from build123d import *

# Parameters (mm, degrees)
BOSS_EXTRUDE1_DEPTH = 247.65
FILLET2_R           = 0.254
FILLET1_R           = 1.27
SKETCH5_W           = 7.112
SKETCH5_H           = 2.54
BOSS_EXTRUDE2_DEPTH = 495.3


with BuildPart() as part:
    # Sketch3 → Boss-Extrude1 (new body, symmetric)
    with BuildSketch(Plane.XY):
        with BuildLine():
            Line((-12.7, 12.7), (-1.796051224, 1.796051224))
            ThreePointArc((-1.796051224, 1.796051224), (-0.972015918, 2.346654013), (0, 2.54))
            Line((0, 2.54), (0, 4.826))
            Line((0, 4.826), (-1.977846327, 4.826))
            ThreePointArc((-1.977846327, 4.826), (-2.949862246, 5.019345987), (-3.773897552, 5.569948776))
            Line((-3.773897552, 5.569948776), (-7.772528286, 9.56857951))
            ThreePointArc((-7.772528286, 9.56857951), (-7.847628361, 9.946133082), (-7.527553898, 10.16))
            Line((-7.527553898, 10.16), (-3.302, 10.16))
            Line((-3.302, 10.16), (-3.302, 12.7))
            Line((-3.302, 12.7), (-12.7, 12.7))
        make_face()
    extrude(amount=BOSS_EXTRUDE1_DEPTH, both=True)

    # Fillet2
    fillet2_edges = [part.edges().sort_by_distance(p)[0] for p in [
        (-3.302, 12.7, 0),
        (-3.302, 10.16, 0),
    ]]
    fillet(fillet2_edges, radius=FILLET2_R)

    # Mirror1: part across plane


with BuildPart() as part_1:
    add(part.part)
    add(part.part.mirror(Plane(origin=(0, 0, 247.65), x_dir=(0, 0, 1), z_dir=(0.707106781, 0.707106781, 0))))

    # Fillet1
    fillet1_edges = [part_1.edges().sort_by_distance(p)[0] for p in [
        (-12.7, 12.7, 0),
    ]]
    fillet(fillet1_edges, radius=FILLET1_R)

    # Mirror2: part across plane


with BuildPart() as part_2:
    add(part_1.part)
    add(part_1.part.mirror(Plane(origin=(0, 0, 247.65), x_dir=(0, 0, 1), z_dir=(0, 1, 0))))

    # Mirror5: part across plane


with BuildPart() as part_3:
    add(part_2.part)
    add(part_2.part.mirror(Plane(origin=(0, 0, 247.65), x_dir=(0, 0, 1), z_dir=(-1, 0, 0))))

    # Sketch5 → Boss-Extrude2 (add, through all)
    with BuildSketch(Plane.XY.offset(247.65)):
        with Locations((0, -11.43)):
            Rectangle(SKETCH5_W, SKETCH5_H)
    extrude(amount=-BOSS_EXTRUDE2_DEPTH)


solid = part_3.part
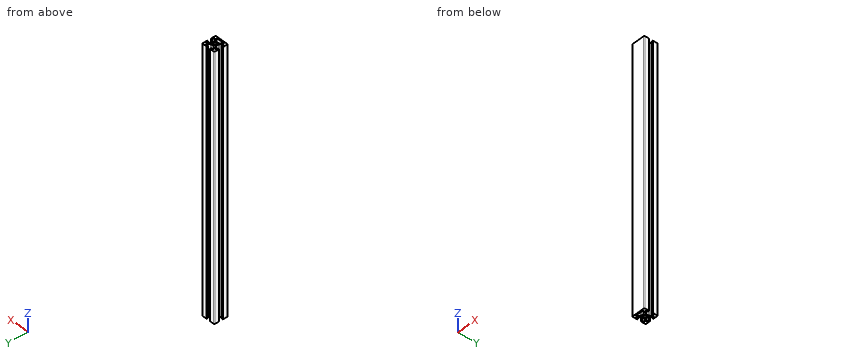
Model file for the job. Use its own axes, mm. Coordinates: 2 decimals unless noted, no trailing zeros. Return JSON: item names as keys, results as strings. Group by question number.
Item 1: Wall check: line 1 along Y through (x, z) = (-11.25, -22.5); line 2 along X through (y, z) = (-9.5, 79.5); line 3 along X through (y, z) = (10, 139.5). Give the ranges that are in metal, low to high. Write a range as [from, to].
Item 2: Saw through at A-A on z = 178.5. State how many separate pieces and enclosed holes the cut face has, then the cut area to 3 significant figures.
Item 3: Flat gauge pins, fed straight in: P1, Ø2, axis at y = 0, z = 70, coming from the -X side; P2, Ø5, axis at x = -7.5, y = -9.5, coming from the -Z side; P3, Ø1.2, axis at x = 0.5, z = 113, coming from the +Y side. Where does each tip first touch, or does it go through?
Values found:
{
 "1": {"line 1": "y = [-12.7, -3.3], [3.3, 12.7]", "line 2": "x = [-12.7, -7.7], [7.7, 12.7]", "line 3": "x = [-12.7, -7.82], [7.82, 12.7]"},
 "2": {"separate pieces": "1", "enclosed holes": "2", "area": "332 mm2"},
 "3": {"P1": "stops at x = -4.83", "P2": "stops at z = -247.65", "P3": "stops at y = 4.83"}
}
